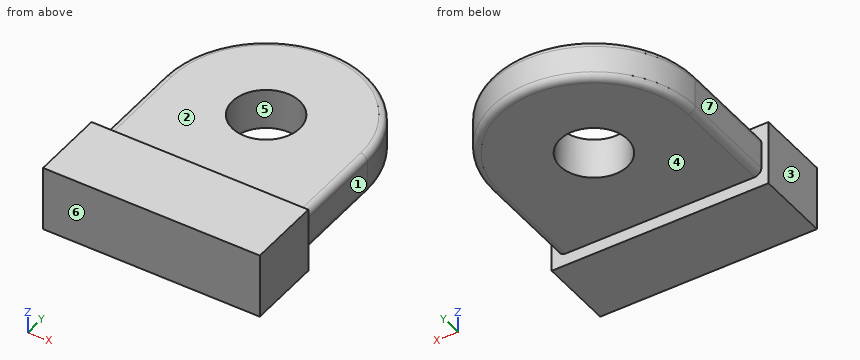
from build123d import *

# Parameters (mm, degrees)
SKETCH1_R           = 5
BOSS_EXTRUDE1_DEPTH = 6
FILLET1_R           = 1
SKETCH2_W           = 32.125499546
SKETCH2_H           = 9.652373674
BOSS_EXTRUDE2_DEPTH = 11


with BuildPart() as part:
    # Sketch1 → Boss-Extrude1 (new body)
    with BuildSketch(Plane.XY):
        with BuildLine():
            Line((-15, 0), (-15, -15))
            Line((-15, -15), (15, -15))
            Line((15, -15), (15, 0))
            ThreePointArc((15, 0), (0, 15), (-15, 0))
        make_face()
        Circle(SKETCH1_R, mode=Mode.SUBTRACT)
    extrude(amount=BOSS_EXTRUDE1_DEPTH)

    # Fillet1
    fillet1_edges = [part.edges().sort_by_distance(p)[0] for p in [
        (15, -7.5, 6),
        (0, 15, 6),
        (15, -7.5, 0),
        (-15, -7.5, 0),
        (0, 15, 0),
        (-15, -7.5, 6),
    ]]
    fillet(fillet1_edges, radius=FILLET1_R)

    # Sketch2 → Boss-Extrude2 (add)
    with BuildSketch(Plane.XZ.offset(15)):
        with Locations((0, 3)):
            Rectangle(SKETCH2_W, SKETCH2_H)
    extrude(amount=BOSS_EXTRUDE2_DEPTH)


solid = part.part
Check sheet for the modelled part. Datum: model origin and axes. Units: mm. Face numbers are marked on the shaded views. A direction names the side the tool comes from. Give positions to 0.01 mm unless a question says otherwise; leave off trailing zeros. Write each loop counter-clockwise with the first axis right and the second up, starting at its lowest first coordinate (ties: lowest second). Pieces come first, ordered by that corner, then holes. Notation, with made-up numbers: (-25, 47.5) -> (-8, 47.5) arc R10 cw to (-8, 60.5) -> close; hole circle Ø11 at (2, -13.5). An arc over 180 degrees is marked (long way). Use one line per item in the form item = value. Start each with the question number.
1. Mould release check, pull along Y, two halves, no side actions. Record for the marked faces 5, 6 and 7: pulls with the +Y half, pulls with the -Y half, needs draft (parallel to the pull), parting line crosses it, or undercut.
2. Section check B-B (z = 3). Record the cut outline in (x, y), and give its area (3 significant figures).
3. Thickness scan on line 1 along Y through (x, z) = (0, 2.7); line 2 along Y through (x, z) = (-1.5, 7.25); line 3 along X through (y, z) = (-9, 1). Record the ranges inside material, lowest first. Write a range as from..to.
4. Go/stop test with flat-tipped pins: P1, Ø3, axis at y = -5.5, z = 2.5, coming from the +X side; P2, Ø12, axis at x = -2.5, y = -3.5, coming from the +Z side; P3, Ø4, axis at x = 8, z = 1, coming from the +Y side. Record where each tip stops, or that it passes through.
5. Section check C-C (y = -12). Record the cut outline in (x, z).
6. Section check A-A (x = 0). Record the cut outline in (y, z).
7. Access from +Z, -Z, +X, -X, +Y, -Y to the whole of each face (thin tool, end or side, straight path). Record for the marked faces 1, 2, 3 and 4.
Conclusion:
q1.face_5 = undercut
q1.face_6 = pulls with the -Y half
q1.face_7 = needs draft
q2.outline = (-16.06, -26) -> (16.06, -26) -> (16.06, -15) -> (15, -15) -> (15, 0) arc R15 ccw to (-15, 0) -> (-15, -15) -> (-16.06, -15) -> close; hole circle Ø10 at (0, 0)
q2.area = 1,080 mm²
q3.line_1 = -26..-5, 5..15
q3.line_2 = -26..-15
q3.line_3 = -15..15
q4.P1 = 15
q4.P2 = 6
q4.P3 = 13.75
q5.outline = (-15, 1) arc R1 ccw to (-14, 0) -> (14, 0) arc R1 ccw to (15, 1) -> (15, 5) arc R1 ccw to (14, 6) -> (-14, 6) arc R1 ccw to (-15, 5) -> close
q6.outline = (-26, -1.83) -> (-15, -1.83) -> (-15, 0) -> (-5, 0) -> (-5, 6) -> (-15, 6) -> (-15, 7.83) -> (-26, 7.83) -> close; (5, 0) -> (14, 0) arc R1 ccw to (15, 1) -> (15, 5) arc R1 ccw to (14, 6) -> (5, 6) -> close
q7.face_1 = +Z, -Z, +X, +Y
q7.face_2 = +Z, +X, -X, +Y
q7.face_3 = +Z, -Z, -X, +Y, -Y
q7.face_4 = -Z, +X, -X, +Y
